```python
from build123d import *

# Parameters (mm, degrees)
SKETCH1_R           = 5
SKETCH1_R_2         = 2.425
BOSS_EXTRUDE1_DEPTH = 7
SKETCH2_W           = 3.5
SKETCH2_H           = 7
BOSS_EXTRUDE3_DEPTH = 1.5
SKETCH4_W           = 7
SKETCH4_H           = 7
SKETCH4_R           = 2.075
BOSS_EXTRUDE4_DEPTH = 5
SKETCH5_R           = 4
CUT_EXTRUDE1_DEPTH  = 0.9


with BuildPart() as part:
    # Sketch1 → Boss-Extrude1 (new body)
    with BuildSketch(Plane(origin=(0, 0, 0), x_dir=(1, 0, 0), z_dir=(0, 1, 0))):
        Circle(SKETCH1_R)
        Circle(SKETCH1_R_2, mode=Mode.SUBTRACT)
    extrude(amount=BOSS_EXTRUDE1_DEPTH)

    # Sketch2 → Boss-Extrude3 (add)
    with BuildSketch(Plane.XY.offset(5)):
        with Locations((-1.75, 3.5)):
            Rectangle(SKETCH2_W, SKETCH2_H)
        with Locations((1.75, 3.5)):
            Rectangle(SKETCH2_W, SKETCH2_H)
    extrude(amount=-BOSS_EXTRUDE3_DEPTH)

    # Sketch4 → Boss-Extrude4 (add)
    with BuildSketch(Plane.XY.offset(5)):
        with Locations((0, 3.5)):
            Rectangle(SKETCH4_W, SKETCH4_H)
        with Locations((0, 3.5)):
            Circle(SKETCH4_R, mode=Mode.SUBTRACT)
    extrude(amount=BOSS_EXTRUDE4_DEPTH)

    # Sketch5 → Cut-Extrude1 (cut)
    with BuildSketch(Plane(origin=(0, 7, 0), x_dir=(1, 0, 0), z_dir=(0, 1, 0))):
        Circle(SKETCH5_R)
    extrude(amount=-CUT_EXTRUDE1_DEPTH, mode=Mode.SUBTRACT)


solid = part.part
```
Check sheet for the modelled part. Datum: model origin and axes. Units: mm. A direction names the side the tool comes from. Give positions to 0.01 mm unless a question says otherwise; leave off trailing zeros. Order: outer loops, then holes, each group sorted by start corner. A loop starts at its lowest first (then second) coordinate and runs counter-clockwise, first axis right, second up. Notation, with made-up numbers: M -6,46.25 L 34,46.25 A30 cw 34,82.25 Z; hole C 48,59.5 d2. An arc over 180 degrees is marked long. Answer in a Markdown table with one row per item. Add a question column.
Q1. Thickness scan on L1, parallel to X at y = 4.75, z = 0 (3 decimals); L2, parallel to X at y = 6.4, z = 0; L3, parallel to Y at x = -1.75, z = 3.5. Record the ranges inside material, lowest first.
Q2. Sectioned sample at A-A, the plane x = 0. Record the boundary of the cut face in (y, z) (3 decimals).
Q3. Sectioned sample at B-B, the plane y = 6.75. Record the boundary of the cut face in (x, z), and give its area (3 significant figures).
Q4. Sectioned sample at C-C, the plane z = 1.75. Record the boundary of the cut face in (x, y), and give its area (3 significant figures).
Q5. Sectioned sample at D-D, the plane z = 7. Record the boundary of the cut face in (x, y) (3 decimals).
Q6. Access from +Z, -Z, +X, -X, +Y, -Y to the whole of each face (thin tool, end or side, straight path). Record for faces 1 (the flat face through (-3.5, 3, 7)), 2 (the cylindrical face through (-0.27, 5.557, 7.465)), 3 (the cylindrical face through (-0.867, 6.556, 3.905)), 4 (the flat face through (3.5, 3, 7)).
Q7. Release check for a two-part mould opening along X. For faces 5 (the flat face through (2, 6.1, 2)), 6 (the flat face through (1, 0, 2.4)), 7 (the cylindrical face through (0, 3, -5)) record: released by +X, released by -X, zero draft, split by the parting line, or undercut.
Q8. Gauge pin test, flat ends, axial feed: pin 1 Ø1 at (x, z) = (-0.5, 3) entering from -Y; pin 2 Ø1.2 at (x, y) = (0.5, 4) entering from +Z; pin 3 Ø4.5 at (x, z) = (0, 0) entering from -Y. Record the tip position at first contact, or that the pin passes through.
Verdict:
| question | item | result |
|---|---|---|
| 1 | L1 | -5 to -2.425, 2.425 to 5 |
| 1 | L2 | -5 to -4, 4 to 5 |
| 1 | L3 | 0 to 6.1 |
| 2 | outline | M 0,-5 L 7,-5 L 7,-4 L 6.1,-4 L 6.1,-2.425 L 0,-2.425 Z; M 0,2.425 L 6.1,2.425 L 6.1,4 L 7,4 L 7,10 L 5.575,10 L 5.575,5 L 1.425,5 L 1.425,10 L 0,10 Z |
| 3 | outline | M -3.5,3.57 A5 ccw long 3.5,3.57 L 3.5,10 L -3.5,10 Z; hole C 0,0 d8 |
| 3 | area | 66.4 mm² |
| 4 | outline | M -4.68,0 L -1.68,0 L -1.68,6.1 L -3.6,6.1 L -3.6,7 L -4.68,7 Z; M 1.68,0 L 4.68,0 L 4.68,7 L 3.6,7 L 3.6,6.1 L 1.68,6.1 Z |
| 4 | area | 38.6 mm² |
| 5 | outline | M -3.5,0 L 3.5,0 L 3.5,7 L -3.5,7 Z; hole C 0,3.5 d4.15 |
| 6 | face 1 | +Z, -X, +Y, -Y |
| 6 | face 2 | +Z |
| 6 | face 3 | +Y |
| 6 | face 4 | +Z, +X, +Y, -Y |
| 7 | face 5 | undercut |
| 7 | face 6 | zero draft |
| 7 | face 7 | split by the parting line |
| 8 | pin 1 | y = 0 |
| 8 | pin 2 | z = 5 |
| 8 | pin 3 | through |
